```python
from build123d import *

# Parameters (mm, degrees)
SKETCH_W   = 115.5
SKETCH_H   = 115.5
SKETCH_R   = 1.5
SKETCH_W_2 = 5.4
SKETCH_H_2 = 5.4
PAD_DEPTH  = 2


with BuildPart() as part:
    # Sketch → Pad (new body)
    with BuildSketch(Plane.XY):
        Rectangle(SKETCH_W, SKETCH_H)
        with Locations((-49.5, 33)):
            Circle(SKETCH_R, mode=Mode.SUBTRACT)
        with Locations((-33, 49.5)):
            Circle(SKETCH_R, mode=Mode.SUBTRACT)
        with Locations((33, 49.5)):
            Circle(SKETCH_R, mode=Mode.SUBTRACT)
        with Locations((49.5, 33)):
            Circle(SKETCH_R, mode=Mode.SUBTRACT)
        with Locations((49.5, -33)):
            Circle(SKETCH_R, mode=Mode.SUBTRACT)
        with Locations((33, -49.5)):
            Circle(SKETCH_R, mode=Mode.SUBTRACT)
        with Locations((-33, -49.5)):
            Circle(SKETCH_R, mode=Mode.SUBTRACT)
        with Locations((-49.5, -33)):
            Circle(SKETCH_R, mode=Mode.SUBTRACT)
        Rectangle(SKETCH_W_2, SKETCH_H_2, mode=Mode.SUBTRACT)
        with Locations((-16.5, 0)):
            Rectangle(SKETCH_W_2, SKETCH_H_2, mode=Mode.SUBTRACT)
        with Locations((-33, 0)):
            Rectangle(SKETCH_W_2, SKETCH_H_2, mode=Mode.SUBTRACT)
        with Locations((16.5, 0)):
            Rectangle(SKETCH_W_2, SKETCH_H_2, mode=Mode.SUBTRACT)
        with Locations((33, 0)):
            Rectangle(SKETCH_W_2, SKETCH_H_2, mode=Mode.SUBTRACT)
        with Locations((0, -16.5)):
            Rectangle(SKETCH_W_2, SKETCH_H_2, mode=Mode.SUBTRACT)
        with Locations((-16.5, -16.5)):
            Rectangle(SKETCH_W_2, SKETCH_H_2, mode=Mode.SUBTRACT)
        with Locations((-33, -16.5)):
            Rectangle(SKETCH_W_2, SKETCH_H_2, mode=Mode.SUBTRACT)
        with Locations((16.5, -16.5)):
            Rectangle(SKETCH_W_2, SKETCH_H_2, mode=Mode.SUBTRACT)
        with Locations((33, -16.5)):
            Rectangle(SKETCH_W_2, SKETCH_H_2, mode=Mode.SUBTRACT)
        with Locations((0, 16.5)):
            Rectangle(SKETCH_W_2, SKETCH_H_2, mode=Mode.SUBTRACT)
        with Locations((-16.5, 16.5)):
            Rectangle(SKETCH_W_2, SKETCH_H_2, mode=Mode.SUBTRACT)
        with Locations((-33, 16.5)):
            Rectangle(SKETCH_W_2, SKETCH_H_2, mode=Mode.SUBTRACT)
        with Locations((16.5, 16.5)):
            Rectangle(SKETCH_W_2, SKETCH_H_2, mode=Mode.SUBTRACT)
        with Locations((33, 16.5)):
            Rectangle(SKETCH_W_2, SKETCH_H_2, mode=Mode.SUBTRACT)
        with Locations((0, 33)):
            Rectangle(SKETCH_W_2, SKETCH_H_2, mode=Mode.SUBTRACT)
        with Locations((-16.5, 33)):
            Rectangle(SKETCH_W_2, SKETCH_H_2, mode=Mode.SUBTRACT)
        with Locations((-33, 33)):
            Rectangle(SKETCH_W_2, SKETCH_H_2, mode=Mode.SUBTRACT)
        with Locations((16.5, 33)):
            Rectangle(SKETCH_W_2, SKETCH_H_2, mode=Mode.SUBTRACT)
        with Locations((33, 33)):
            Rectangle(SKETCH_W_2, SKETCH_H_2, mode=Mode.SUBTRACT)
        with Locations((0, -33)):
            Rectangle(SKETCH_W_2, SKETCH_H_2, mode=Mode.SUBTRACT)
        with Locations((-16.5, -33)):
            Rectangle(SKETCH_W_2, SKETCH_H_2, mode=Mode.SUBTRACT)
        with Locations((-33, -33)):
            Rectangle(SKETCH_W_2, SKETCH_H_2, mode=Mode.SUBTRACT)
        with Locations((16.5, -33)):
            Rectangle(SKETCH_W_2, SKETCH_H_2, mode=Mode.SUBTRACT)
        with Locations((33, -33)):
            Rectangle(SKETCH_W_2, SKETCH_H_2, mode=Mode.SUBTRACT)
    extrude(amount=PAD_DEPTH)


solid = part.part
```
The model under review builds one solid part; all positions refer to its coordinate system, in mm. Coordinates: 2 decimals unless noted, no trailing zeros. Write each loop counter-clockwise with the first axis right and the second up, starting at its lowest first coordinate (ties: lowest second). Pieces come first, ordered by that corner, then holes. Notation, with made-up numbers: (-39.75, -27) -> (10.25, -27) arc R23 cw to (10.25, 8) -> close; hole circle Ø10 at (64, 48). An arc over 180 degrees is marked (long way). One line per item, written item: value. Start each with the question number.
Q1. Add section C-C, the plane x = 49.5. Give the boundary of the cut face in (y, z).
Q2. Add section B-B, the plane y = 16.5. Give the boundary of the cut face in (x, z), then the cut area to 3 significant figures.
Q3. Add section A-A, the plane x = -33. Count the separate pieces of the cut face and the enclosed holes in it, then the cut area to 3 significant figures.
Q4. The part is to be moulded in two halves that separate along X. For faces 1 (the face through (-0.8, 13.6, 2)), 2 (the face through (48.3, 32.1, 1)), say which applies: +X half, -X half, draft (parallel to the pull), parting line (faces both ways), or undercut.
Q5. To check wall thickness, follow probe 1 along Y at (x, z) = (49.5, 0.4); probe 2 along X at (y, z) = (-14, 1.1). State the ranges of each line that lie inside material, in increasing order.
Response:
1. outline: (-57.75, 0) -> (-34.5, 0) -> (-34.5, 2) -> (-57.75, 2) -> close; (-31.5, 0) -> (31.5, 0) -> (31.5, 2) -> (-31.5, 2) -> close; (34.5, 0) -> (57.75, 0) -> (57.75, 2) -> (34.5, 2) -> close
2. outline: (-57.75, 0) -> (-35.7, 0) -> (-35.7, 2) -> (-57.75, 2) -> close; (-30.3, 0) -> (-19.2, 0) -> (-19.2, 2) -> (-30.3, 2) -> close; (-13.8, 0) -> (-2.7, 0) -> (-2.7, 2) -> (-13.8, 2) -> close; (2.7, 0) -> (13.8, 0) -> (13.8, 2) -> (2.7, 2) -> close; (19.2, 0) -> (30.3, 0) -> (30.3, 2) -> (19.2, 2) -> close; (35.7, 0) -> (57.75, 0) -> (57.75, 2) -> (35.7, 2) -> close
2. area: 177 mm²
3. separate pieces: 8
3. enclosed holes: 0
3. area: 165 mm²
4. face 1: draft
4. face 2: undercut
5. probe 1: -57.75 to -34.5, -31.5 to 31.5, 34.5 to 57.75
5. probe 2: -57.75 to -35.7, -30.3 to -19.2, -13.8 to -2.7, 2.7 to 13.8, 19.2 to 30.3, 35.7 to 57.75
